from build123d import *

# Parameters (mm, degrees)
PAD_DEPTH                  = 5
POCKET_DEPTH               = 416.682466
PAD001_DEPTH               = 1
PAD001_MIRRORED002_2_DEPTH = 1
FILLET_R                   = 2
BODY_PLACEMENT_ANGLE       = 180


with BuildPart() as part:
    # Sketch → Revolution (revolve)
    with BuildSketch(Plane.XZ):
        Polygon((2.5, 53), (55, 4), (59.5, 4), (59.5, 11), (64, 11), (64, 0), (55, 0), (2.5, 48), align=None)
    revolve(axis=Axis((0, 0, 0), (0, 0, 1)))

    # Sketch001 → Pad (new body, symmetric)
    with BuildSketch(Plane.XZ):
        Polygon((9, 45), (20, 55), (20, 87), (30, 87), (34, 23), align=None)
    pad = extrude(amount=PAD_DEPTH, both=True)

    # Mirrored: Pad across Sketch001 V_Axis
    add(pad.mirror(Plane(origin=(0, 0, 0), x_dir=(0, -1, 0), z_dir=(1, 0, 0))))

    # Sketch003 (on DatumPlane) → Pocket (cut, through all)
    with BuildSketch(Plane.XY.offset(72)):
        Polygon((27, 0), (26, 1.732051), (24, 1.732051), (23, 0), (24, -1.732051), (26, -1.732051), align=None)
    pocket = extrude(amount=POCKET_DEPTH, mode=Mode.SUBTRACT)

    # Mirrored001: Pocket across Sketch003 V_Axis
    add(pocket.mirror(Plane(origin=(0, 0, 72), x_dir=(0, 0, 1), z_dir=(1, 0, 0))), mode=Mode.SUBTRACT)

    # Sketch004 (on DatumPlane) → Pad001 (join, symmetric)
    with BuildSketch(Plane.YZ.offset(-25)):
        Polygon((5, 87), (26, 20), (4, 30), (4, 86), align=None)
    pad001 = extrude(amount=PAD001_DEPTH, both=True)

    # Sketch004 Mirrored002 2 → Pad001 Mirrored002 2 (add, symmetric)
    with BuildSketch(Plane(origin=(-25, 0, 0), x_dir=(0, -1, 0), z_dir=(-1, 0, 0))):
        Polygon((5, 87), (26, 20), (4, 30), (4, 86), align=None)
    pad001_mirrored002_2 = extrude(amount=-PAD001_MIRRORED002_2_DEPTH, both=True)

    # Mirrored003: Pad001, Pad001 Mirrored002 2 across YZ
    add(pad001.mirror(Plane.YZ))
    add(pad001_mirrored002_2.mirror(Plane.YZ))

    # Fillet
    fillet_edges = [part.edges().sort_by_distance(p)[0] for p in [
        (-31.991421, -5, 55.137271),
        (-31.991421, 5, 55.137271),
        (31.991421, -5, 55.137271),
        (31.991421, 5, 55.137271),
        (-20, 5, 71),
        (-20, -5, 71),
        (-14.709357, -5, 50.190324),
        (14.709357, -5, 50.190324),
        (20, -5, 71),
        (-2.5, 0, 48),
        (-59.5, 0, 11),
        (20, 5, 71),
        (14.709357, 5, 50.190324),
        (-14.709357, 5, 50.190324),
    ]]
    fillet(fillet_edges, radius=FILLET_R)


with BuildPart() as part_1:
    # Body placement: moved
    add(part.part.rotate(Axis((0, 0, 0), (1, 0, 0)), BODY_PLACEMENT_ANGLE))


solid = part_1.part
Model file for the job. Use its own axes, mm. A direction names the side the tool comes from. Give positions to 0.01 mm unless a question says otherwise; leave off trailing zeros. Put each result on its own line as item: value. Start each with the question number.
(1) Pin check, flat tips, straight feed: pin 1 Ø1.5 at (x, z) = (11, -35.5) entering from +Y; pin 2 Ø0.6 at (x, z) = (-24.5, -82.5) entering from +Y; pin 3 Ø22.5 at (y, z) = (16.5, -65) entering from -X; pin 4 Ø1.7 at (x, y) = (-25.5, 1) entering from -Z. Stop position of each tip, or through.
(2) Pull direction Y, two halves, no side cores. Call faces 1 (the face through (-26, 11, -47)), 2 (the face through (28, 5, -50)), 3 (the face through (25, 0, -72)): released by +Y, released by -Y, zero draft, split by the parting line, or undercut.
(3) Tool access for faces 4 (the face through (24.986, -15.155, -54.599)), 5 (the face through (-24.986, 15.155, -54.599)), 6 (the face through (-25, 0, -72)): list every direction of +Z, -Z, +X, -X, +Y, -Y with a clear straight run to the whole face (end or side of a thin tool).
(4) Band-saw the part on A-A on z = -50.5. Count the separate pieces of the cut face and the enclosed holes in it, then the cut area to 3 significant figures.
(5) Drill centre lines: L1, parallel to X at y = 0, z = -6.9; L2, parallel to Y at x = 0, z = -50.7; L3, parallel to Y at x = 0, z = -5.85. Where is each one in solid material? Low to high. Write a range as [from, to].
Results below:
1. pin 1: stops at y = 19.21
1. pin 2: stops at y = 6.5
1. pin 3: stops at x = -26
1. pin 4: stops at z = -87
2. face 1: zero draft
2. face 2: released by +Y
2. face 3: undercut
3. face 4: -Z, +X, -Y
3. face 5: -Z, -X, +Y
3. face 6: -Z
4. separate pieces: 3
4. enclosed holes: 1
4. area: 492 mm2
5. L1: x = [-64, -59.5], [-51.89, -47.45], [47.45, 51.89], [59.5, 64]
5. L2: y = [-4.96, -2.5], [2.5, 4.96]
5. L3: y = [-64, -59.5], [-53.02, -48.6], [48.6, 53.02], [59.5, 64]
